Can you work these out from the model? Positions are in its coordinate system, mm. A direction names the side the tool comes from. Give positions to 0.01 mm unless a question says otherwise; leave off trailing zeros. Write each loop counter-clockwise with the first axis right and the second up, starting at its lowest first coordinate (ties: lowest second). Pieces come first, ordered by that corner, then holes. Notation, with made-up numbers: M -34,75 L 20,75 A4 cw 20,81 Z; hole C -0.5,35.5 d9. An arc over 180 degrees is marked long. Use CSV: the item, a comma, the result in double quotes. Start each with the question number.
from build123d import *

# Parameters (mm, degrees)
SKETCH1_W                = 100
SKETCH1_H                = 120
BOSS_EXTRUDE1_DEPTH      = 5
SKETCH2_W                = 100
SKETCH2_H                = 2
BOSS_EXTRUDE2_DEPTH      = 45
BOSS_EXTRUDE3_DEPTH      = 40
BOSS_EXTRUDE3_DEPTH_BACK = 60
SKETCH3_W                = 100
SKETCH3_H                = 5
SKETCH6_W                = 100
SKETCH6_H                = 5
BOSS_EXTRUDE4_DEPTH      = 15
SKETCH7_W                = 100
SKETCH7_H                = 5
BOSS_EXTRUDE5_DEPTH      = 45
SKETCH8_R                = 16
SKETCH8_R_2              = 1.5
CUT_EXTRUDE1_DEPTH       = 93.736184955
SKETCH10_R               = 5.1
CUT_EXTRUDE2_DEPTH       = 93.736184955


with BuildPart() as part:
    # Sketch1 → Boss-Extrude1 (new body)
    with BuildSketch(Plane.XY):
        Rectangle(SKETCH1_W, SKETCH1_H)
    extrude(amount=BOSS_EXTRUDE1_DEPTH)

    # Sketch2 → Boss-Extrude2 (add)
    with BuildSketch(Plane.XY.offset(5)):
        with Locations((0, 19)):
            Rectangle(SKETCH2_W, SKETCH2_H)
    extrude(amount=BOSS_EXTRUDE2_DEPTH)

    # Sketch3 → Boss-Extrude3 (add, two sides: drawn at the far end of the back side and taken through both)
    with BuildSketch(Plane(origin=(0, 20, 0), x_dir=(1, 0, 0), z_dir=(0, 1, 0)).offset(-BOSS_EXTRUDE3_DEPTH_BACK)):
        with Locations((0, -47.5)):
            Rectangle(SKETCH3_W, SKETCH3_H)
    extrude(amount=BOSS_EXTRUDE3_DEPTH + BOSS_EXTRUDE3_DEPTH_BACK)

    # Sketch6 → Boss-Extrude4 (add)
    with BuildSketch(Plane.XZ.offset(40)):
        with Locations((0, 47.5)):
            Rectangle(SKETCH6_W, SKETCH6_H)
        with Locations((0, 2.5)):
            Rectangle(SKETCH6_W, SKETCH6_H)
    extrude(amount=BOSS_EXTRUDE4_DEPTH)

    # Sketch7 → Boss-Extrude5 (add)
    with BuildSketch(Plane.XY.offset(5)):
        with Locations((0, -57.5)):
            Rectangle(SKETCH7_W, SKETCH7_H)
    extrude(amount=BOSS_EXTRUDE5_DEPTH)

    # Sketch8 → Cut-Extrude1 (cut, through all)
    with BuildSketch(Plane.XY.offset(50)):
        with Locations((0, -22.5)):
            Circle(SKETCH8_R)
        with Locations((0, 2.5)):
            Circle(SKETCH8_R_2)
        with Locations((21.650635095, -10)):
            Circle(SKETCH8_R_2)
        with Locations((21.650635095, -35)):
            Circle(SKETCH8_R_2)
        with Locations((0, -47.5)):
            Circle(SKETCH8_R_2)
        with Locations((-21.650635095, -35)):
            Circle(SKETCH8_R_2)
        with Locations((-21.650635095, -10)):
            Circle(SKETCH8_R_2)
    extrude(amount=-CUT_EXTRUDE1_DEPTH, mode=Mode.SUBTRACT)

    # Sketch10 → Cut-Extrude2 (cut, through all)
    with BuildSketch(Plane.XY.offset(50)):
        with Locations((-43, 40)):
            Circle(SKETCH10_R)
        with Locations((43, 40)):
            Circle(SKETCH10_R)
    extrude(amount=-CUT_EXTRUDE2_DEPTH, mode=Mode.SUBTRACT)


solid = part.part
(1) I want a section at C-C (z = 10). Write out the boundary of the cut face in (x, y).
(2) Thinking about a two-plate mould opening in Z: for faces 1 (the face through (-12, -10, 5)), 2 (the face through (0, 1, 48)), which applies, released by +Z, released by -Z, zero draft, split by the parting line, or undercut?
(3) I want a section at B-B (y = 2.5). Write out the boundary of the cut face in (x, z).
(4) Please list where these lines run through material, in increasing order: L1, parallel to Z at x = -19.5, y = 1.5; L2, parallel to Y at x = 3, z = 23.5; L3, parallel to Y at x = 0, z = 3.35. Write a range as [from, to].
(5) Which directions (+Z, -Z, +X, -X, +Y, -Y) give clear straight access to the entire face, cutting with the end or side of a thin tool? Please do faces 3 (the face through (-12, -10, 45)), 4 (the face through (-3.47, -38.12, 2.53)).
(6) Will this pin go through, and if not, where does the flat tip stop? pin 1 Ø8 at (x, z) = (-5.5, 30) entering from +Y.
(7) I want a section at A-A (x = -43). Write out the boundary of the cut face in (y, z).
(8) I want a section at D-D (y = 40). Write out the boundary of the cut face in (x, z), and give its area (3 significant figures).
Geometry results:
1,outline,"M -50,-60 L 50,-60 L 50,-55 L -50,-55 Z; M -50,18 L 50,18 L 50,20 L -50,20 Z"
2,face 1,"undercut"
2,face 2,"zero draft"
3,outline,"M -50,0 L -1.5,0 L -1.5,5 L -50,5 Z; M -50,45 L -1.5,45 L -1.5,50 L -50,50 Z; M 1.5,0 L 50,0 L 50,5 L 1.5,5 Z; M 1.5,45 L 50,45 L 50,50 L 1.5,50 Z"
4,L1,"z = [0, 5], [45, 50]"
4,L2,"y = [-60, -55], [18, 20]"
4,L3,"y = [-60, -49], [-46, -38.5], [-6.5, 1], [4, 60]"
5,face 3,"+X, -X"
5,face 4,"+Z, -Z"
6,pin 1,"stops at y = 20"
7,outline,"M -60,0 L 34.9,0 L 34.9,5 L 20,5 L 20,45 L 34.9,45 L 34.9,50 L -60,50 Z; M 45.1,0 L 60,0 L 60,5 L 45.1,5 Z; M 45.1,45 L 60,45 L 60,50 L 45.1,50 Z; hole M -55,5 L 18,5 L 18,45 L -55,45 Z"
8,outline,"M -50,0 L -48.1,0 L -48.1,5 L -50,5 Z; M -50,45 L -48.1,45 L -48.1,50 L -50,50 Z; M -37.9,0 L 37.9,0 L 37.9,5 L -37.9,5 Z; M -37.9,45 L 37.9,45 L 37.9,50 L -37.9,50 Z; M 48.1,0 L 50,0 L 50,5 L 48.1,5 Z; M 48.1,45 L 50,45 L 50,50 L 48.1,50 Z"
8,area,"796 mm2"
